For this review, take the finished solid that the model builds, in its own axes (mm). Give positions to 0.01 mm unless a question says otherwise; leave off trailing zeros. Write each loop counter-clockwise with the first axis right and the second up, starting at its lowest first coordinate (ties: lowest second). Pieces come first, ordered by that corner, then holes. Notation, with made-up numbers: (-22.75, -19) -> (13.25, -19) arc R10 cw to (13.25, -9) -> close; hole circle Ø7 at (-10, -7). An arc over 180 degrees is marked (long way). Write item = value, one per line.
```python
from build123d import *

# Parameters (mm, degrees)
SKETCH1_R           = 12.7
BOSS_EXTRUDE1_DEPTH = 685.8
CUT_EXTRUDE1_START  = 1.1684
SKETCH2_R           = 12.7
SKETCH2_R_2         = 11.938
CUT_EXTRUDE1_DEPTH  = 1.1684


with BuildPart() as part:
    # Sketch1 → Boss-Extrude1 (new body)
    with BuildSketch(Plane(origin=(0, 0, 0), x_dir=(0, 0, -1), z_dir=(1, 0, 0))):
        Circle(SKETCH1_R)
    extrude(amount=BOSS_EXTRUDE1_DEPTH)

    # Sketch2 → Cut-Extrude1 (cut)
    with BuildSketch(Plane.ZY.offset(-10.16).offset(CUT_EXTRUDE1_START)):
        Circle(SKETCH2_R)
        Circle(SKETCH2_R_2, mode=Mode.SUBTRACT)
    cut_extrude1 = extrude(amount=-CUT_EXTRUDE1_DEPTH, mode=Mode.SUBTRACT)

    # Mirror1: Cut-Extrude1 across plane
    add(cut_extrude1.mirror(Plane.ZY.offset(-342.9)), mode=Mode.SUBTRACT)


solid = part.part
```
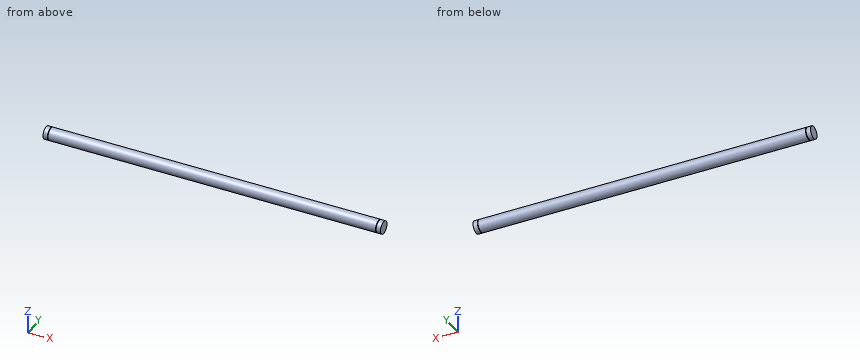
(1) Take a section at C-C (z = -6.25). Write out the cut boundary in (x, y).
Answers below:
outline = (0, -11.06) -> (8.99, -11.06) -> (8.99, -10.17) -> (10.16, -10.17) -> (10.16, -11.06) -> (675.64, -11.06) -> (675.64, -10.17) -> (676.81, -10.17) -> (676.81, -11.06) -> (685.8, -11.06) -> (685.8, 11.06) -> (676.81, 11.06) -> (676.81, 10.17) -> (675.64, 10.17) -> (675.64, 11.06) -> (10.16, 11.06) -> (10.16, 10.17) -> (8.99, 10.17) -> (8.99, 11.06) -> (0, 11.06) -> close
(2) For pin 1 (2 mm diameter, centred on x = 278.5, z = -7, fed in from -Y); pin 2 (1 mm diameter, centred on x = 452.5, z = 5.5, fed in from -Y); pin 3 (1 mm diameter, centred on x = 158, y = -6, fed in from -Z), all flat-tipped, find the tip position at first contact; note any pin that passes through.
Answers below:
pin_1 = -11.19
pin_2 = -11.67
pin_3 = -11.45
(3) To check wall thickness, follow probe 1 along X at (y, z) = (11, 5); probe 2 along Y at (x, z) = (164.5, 1.75); probe 3 along Z at (x, y) = (632, -6.75). State the ranges of each line that lie inside material, in increasing order.
Answers below:
probe_1 = 0 to 8.99, 10.16 to 675.64, 676.81 to 685.8
probe_2 = -12.58 to 12.58
probe_3 = -10.76 to 10.76
(4) Take a section at B-B (x = 559). Write out the cut boundary in (y, z), plus the area to 3 significant figures.
Answers below:
outline = circle Ø25.4 at (0, 0)
area = 507 mm^2
(5) Take a section at A-A (y = 6). Write out the cut boundary in (x, z).
Answers below:
outline = (0, -11.19) -> (8.99, -11.19) -> (8.99, -10.32) -> (10.16, -10.32) -> (10.16, -11.19) -> (675.64, -11.19) -> (675.64, -10.32) -> (676.81, -10.32) -> (676.81, -11.19) -> (685.8, -11.19) -> (685.8, 11.19) -> (676.81, 11.19) -> (676.81, 10.32) -> (675.64, 10.32) -> (675.64, 11.19) -> (10.16, 11.19) -> (10.16, 10.32) -> (8.99, 10.32) -> (8.99, 11.19) -> (0, 11.19) -> close
